Here's how the part is built. I have some questions about the finished solid (model axes, mm). Round coordinates to 2 decimals unless told otherwise and drop trailing zeros. Order: outer loops, then holes, each group sorted by start corner. A loop starts at its lowest first (then second) coordinate and runs counter-clockwise, first axis right, second up. Notation, with made-up numbers: (-21.75, -26) -> (18.25, -26) arc R32 cw to (18.25, 0) -> close; hole circle Ø8 at (11.25, -9.75). An arc over 180 degrees is marked (long way). Use a Markdown table: item, result. Add a question column.
(1) I want a section at B-B, the plane x = 132. Please give me the cut outline in (y, z), then the cut area to 3 significant figures.
(2) I want a section at C-C, the plane z = 2. Please give me the cut outline in (x, y).
(3) I'm going to push flat-ended pins straight in: P1, Ø3, axis at y = 24, z = 2.5, coming from the -X side; P2, Ø2, axis at x = 130.5, z = 3.5, coming from the -Y side; P3, Ø2, axis at y = 13.5, z = 6.5, coming from the -X side. Where does each tip first touch, or does it pass through?
(4) I want a section at A-A, the plane y = 32. Please give me the cut outline in (x, z), then the cut area to 3 significant figures.
(5) If I drill on probe 1 along Z at (x, y) = (138.5, 45.5); probe 2 along X at (y, z) = (20.5, 5); probe 3 along X at (y, z) = (19.5, 1.75), over which ranges is the centre line in solid material (lowest first)?
(6) Thinking about a two-plate mould opening in X: for faces 1 (the face through (108.726, 67.412, 4.43)), 2 (the face through (110.338, 31.571, 4.238)), 3 (the face through (137, 33, 1)), which applies, pulls with the +X half, pulls with the -X half, needs draft (parallel to the pull), parting line crosses it, or undercut?
from build123d import *

# Parameters (mm, degrees)
IZIM1_W                     = 40
IZIM1_H                     = 96
IZIM1_W_2                   = 15
IZIM1_R                     = 1.5
Y_KSEKLIK_EKSTR_ZYON2_DEPTH = 1
IZGIDEN_START               = 43.181135212
IZGIDEN_B_KME3_OUTLINE_R    = 1.5
IZGIDEN_B_KME3_DEPTH        = 3.071295426
IZGIDEN_START_2             = -15.757423971
IZGIDEN_B_KME3_2_DEPTH      = 96
IZGIDEN_B_KME3_3_DEPTH      = 96
IZGIDEN_START_3             = 48
IZGIDEN_B_KME3_4_OUTLINE_R  = 1.5
IZGIDEN_B_KME3_4_DEPTH      = 2.471326215


with BuildPart() as part:
    # Çizim1 → Yükseklik-Ekstrüzyon2 (new body)
    # profile 1 of 2: a face of its own
    with BuildSketch(Plane.XY):
        with Locations((137.175270501, 32.242576029)):
            Rectangle(IZIM1_W, IZIM1_H)
    # profile 2 of 2: a face of its own
    with BuildSketch(Plane.XY):
        with Locations((109.675270501, 32.242576029)):
            Rectangle(IZIM1_W_2, IZIM1_H)
        with Locations((107.175270501, -4.257423971)):
            Circle(IZIM1_R, mode=Mode.SUBTRACT)
        with Locations((107.175270501, 68.742576029)):
            Circle(IZIM1_R, mode=Mode.SUBTRACT)
    extrude(amount=Y_KSEKLIK_EKSTR_ZYON2_DEPTH)

    # Çizgiden Bükme3: read off the stored shape, not the designer's step
    # Çizgiden Bükme3 outline → Çizgiden Bükme3 (cut)
    with BuildSketch(Plane(origin=(0, 0, 0), x_dir=(0.9063077870366497, 0, -0.42261826174069983), z_dir=(0.4226182617406999, 0, 0.9063077870366498)).offset(IZGIDEN_START)):
        with Locations((95.975461344, -4.257423971)):
            Circle(IZGIDEN_B_KME3_OUTLINE_R)
        with Locations((95.975461344, 68.742576029)):
            Circle(IZGIDEN_B_KME3_OUTLINE_R)
    extrude(amount=IZGIDEN_B_KME3_DEPTH, mode=Mode.SUBTRACT)

    # izgiden B_kme3 2 outline → izgiden B_kme3 2 (cut)
    with BuildSketch(Plane(origin=(0, 0, 0), x_dir=(1, 0, 0), z_dir=(0, 1, 0)).offset(IZGIDEN_START_2)):
        with BuildLine():
            Line((102.175270501, -1), (114.91462349, -1))
            Line((114.91462349, -1), (116.657283212, -0.187384426))
            ThreePointArc((116.657283212, -0.187384426), (117.069640507, -0.047407986), (117.502519735, 0))
            Line((117.502519735, 0), (102.175270501, 0))
            Line((102.175270501, 0), (102.175270501, -1))
        make_face()
    extrude(amount=IZGIDEN_B_KME3_2_DEPTH, mode=Mode.SUBTRACT)

    # izgiden B_kme3 3 outline → izgiden B_kme3 3 (add)
    with BuildSketch(Plane(origin=(0, 0, 0), x_dir=(1, 0, 0), z_dir=(0, 1, 0)).offset(IZGIDEN_START_2)):
        with BuildLine():
            Line((103.359254936, -6.388356849), (103.781873198, -7.294664636))
            Line((103.781873198, -7.294664636), (117.079901474, -1.093692213))
            ThreePointArc((117.079901474, -1.093692213), (117.286080121, -1.023703993), (117.502519735, -1))
            Line((117.502519735, -1), (114.91462349, -1))
            Line((114.91462349, -1), (103.359254936, -6.388356849))
        make_face()
    extrude(amount=IZGIDEN_B_KME3_3_DEPTH)

    # izgiden B_kme3 4 outline → izgiden B_kme3 4 (cut)
    with BuildSketch(Plane(origin=(0, 0, 0), x_dir=(0.9063077870366497, 0, -0.42261826174069983), z_dir=(0.4226182617406999, 0, 0.9063077870366498)).offset(IZGIDEN_START_3)):
        with Locations((95.975461344, -4.257423971)):
            Circle(IZGIDEN_B_KME3_4_OUTLINE_R)
        with Locations((95.975461344, 68.742576029)):
            Circle(IZGIDEN_B_KME3_4_OUTLINE_R)
    extrude(amount=IZGIDEN_B_KME3_4_DEPTH, mode=Mode.SUBTRACT)


solid = part.part
Taken from the geometry:
| question | item | result |
|---|---|---|
| 1 | outline | (-15.76, 0) -> (80.24, 0) -> (80.24, 1) -> (-15.76, 1) -> close |
| 1 | area | 96.0 mm2 |
| 2 | outline | (112.77, -15.76) -> (115.14, -15.76) -> (115.14, 80.24) -> (112.77, 80.24) -> close |
| 3 | P1 | stops at x = 108.48 |
| 3 | P2 | passes through |
| 3 | P3 | stops at x = 103.36 |
| 4 | outline | (103.36, 6.39) -> (116.66, 0.19) arc R2 ccw to (117.5, 0) -> (157.18, 0) -> (157.18, 1) -> (117.5, 1) arc R1 cw to (117.08, 1.09) -> (103.78, 7.29) -> close |
| 4 | area | 55.0 mm2 |
| 5 | probe 1 | z = 0 to 1 |
| 5 | probe 2 | x = 106.34 to 108.7 |
| 5 | probe 3 | x = 113.31 to 115.67 |
| 6 | face 1 | undercut |
| 6 | face 2 | pulls with the +X half |
| 6 | face 3 | needs draft |
